CAD build for the part. Positions are in the model's coordinates, mm. Face numbers are marked on the shaded views. A direction names the side the tool comes from. Round coordinates to 2 decimals unless told otherwise and drop trailing zeros. Loops run counter-clockwise (first coordinate to the right, second up) from the corner with the lowest first, then second, coordinate; pieces in that order, holes last.
Autodesk Inventor part; units mm, degrees
ref_plane "Start plane" through (0, 0, 15.875) normal (0, 0, 1) x (1, 0, 0)
ref_plane "End plane" through (0, 0, 98.425) normal (0, 0, 1) x (1, 0, 0)
ref_plane "Work Plane4" through (-9.525, 101.6003, 15.875) normal (0, 0, -1) x (-1, 0, 0)
ref_plane "Start plane" through (0, 0, 15.875) normal (0, 0, 1) x (1, 0, 0)
ref_plane "End plane" through (0, 0, 98.425) normal (0, 0, 1) x (1, 0, 0)
sketch "Sketch" plane through (0, 0, 0) normal (0, 0, 1) x (1, 0, 0)
  line L0 (-15.875, -9.525) -> (-15.875, 9.525)
  line L1 (-9.525, 15.875) -> (9.525, 15.875)
  line L2 (15.875, 9.525) -> (15.875, -9.525)
  line L3 (9.525, -15.875) -> (-9.525, -15.875)
  arc A0 (-15.875, -9.525) -> (-9.525, -15.875) centre (-9.525, -9.525) ccw
  arc A1 (-9.525, 15.875) -> (-15.875, 9.525) centre (-9.525, 9.525) ccw
  arc A2 (15.875, 9.525) -> (9.525, 15.875) centre (9.525, 9.525) ccw
  arc A3 (9.525, -15.875) -> (15.875, -9.525) centre (9.525, -9.525) ccw
  arc A4 (-9.525, 12.7) -> (-12.7, 9.525) centre (-9.525, 9.525) ccw
  line L4 (-9.525, 12.7) -> (9.525, 12.7)
  arc A5 (12.7, 9.525) -> (9.525, 12.7) centre (9.525, 9.525) ccw
  line L5 (12.7, 9.525) -> (12.7, -9.525)
  arc A6 (9.525, -12.7) -> (12.7, -9.525) centre (9.525, -9.525) ccw
  line L6 (9.525, -12.7) -> (-9.525, -12.7)
  arc A7 (-12.7, -9.525) -> (-9.525, -12.7) centre (-9.525, -9.525) ccw
  line L7 (-12.7, -9.525) -> (-12.7, 9.525)
  line L8 (0, 24.0662) -> (0, -24.0662) construction
  line L9 (-24.0662, 0) -> (24.0662, 0) construction
  dimension "d10" = 31.75
  dimension "d11" = 31.75
  dimension "d12" = 3.175
  dimension "d15" = 15.875
  dimension "d16" = 15.875
  dimension "d17" = 6.35
extrude "Body" add sketch "Sketch" along normal up to surface (82.55 mm away) from surface at 15.875
sketch "Sketch3" plane through (0, 0, 0) normal (0, 0, 1) x (1, 0, 0)
  line L0 (0, 0) -> (10, 0)
ref_plane "Work Plane3" through (0, 0, 0) normal (0, -1, 0) x (1, 0, 0)
sketch "Sketch4" plane through (0, 0, 0) normal (0, -1, 0) x (1, 0, 0)
  line L0 (-2, 15.875) -> (12, 15.875)
  line L1 (-2, 98.425) -> (12, 98.425)
  dimension "d19" = 82.55
ref_plane "Work Plane4" through (-9.525, 101.6003, 15.875) normal (0, 0, -1) x (-1, 0, 0)
split "Split1" plane through (-9.525, 101.6003, 15.875) removes the side toward (0, 0, -1)
ref_plane "Work Plane5" through (9.525, 101.6003, 98.425) normal (0, 0, 1) x (1, 0, 0)
split "Split2" plane through (9.525, 101.6003, 98.425) removes the side toward (0, 0, 1)
equation "\"d10\" = G_H"
equation "\"d11\" = G_W"
equation "\"d12\" = G_T"
equation "\"d15\" = 0.5 * d10"
equation "\"d16\" = 0.5 * d11"
equation "\"d17\" = G_IR"
equation "\"d3\" = G_L"
equation "\"G_W\" = 31.75"
equation "\"G_H\" = 31.75"
equation "\"G_T\" = 3.175"
equation "\"G_IR\" = 6.35"
equation "\"G_L\" = d19"
equation "\"G_OFFSET_START\" = -15.875"
equation "\"G_OFFSET_END\" = -15.875"
equation "\"d13\" = -G_OFFSET_START"
equation "\"d14\" = G_OFFSET_END + B_L"
equation "\"B_L\" = 114.3"
properties part number "AISC HSS - 1-1/4x1-1/4x1/8 - 3.25" material "Steel, Mild"
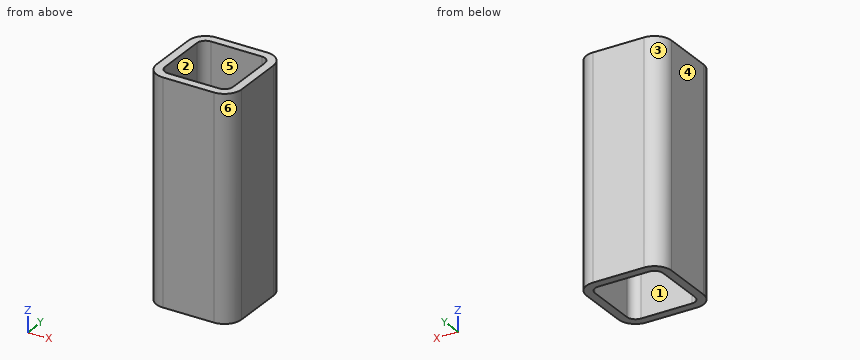
Item 1: Mould opens along Y. For the marked faces 1, 2, 3 and 4 say: released by +Y, released by -Y, zero draft, split by the parting line, or undercut.
Verdict:
face 1: undercut
face 2: undercut
face 3: released by +Y
face 4: zero draft
Item 2: Flat gauge pins, fed straight in: P1, Ø2, axis at x = -12, z = 60, coming from the -Y side; P2, Ø3, axis at y = -12, z = 63, coming from the +X side; P3, Ø4, axis at y = 12, z = 83, coming from the -X side; P4, Ø3, axis at x = 8, y = -10.5, coming from the +Z side. Where does each tip first touch, or does it go through?
Verdict:
P1: stops at y = -15.7
P2: stops at x = 15.8
P3: stops at x = -15.86
P4: passes through
Item 3: Cut at B-B (x = -11.5). List the corners of the cut face in (y, z) (3 decimals).
Verdict:
outline: (-15.56, 15.875) - (-12.011, 15.875) - (-12.011, 98.425) - (-15.56, 98.425) - close; (12.011, 15.875) - (15.56, 15.875) - (15.56, 98.425) - (12.011, 98.425) - close
Item 4: 3-axis set-ups, long thin cutter, end or side, ignore diameter. For the marked faces 5 and 6: which of +Z, -Z, +X, -X, +Y, -Y reach the whole face in a straight line?
Verdict:
face 5: +Z, -Z
face 6: +Z, -Z, +X, -Y
Item 5: Cut at C-C (z = 60). List the corners of the cut face in (x, y) (3 decimals), plus the area to 3 significant figures.
Verdict:
outline: (-15.875, -9.525) arc R6.35 ccw to (-9.525, -15.875) - (9.525, -15.875) arc R6.35 ccw to (15.875, -9.525) - (15.875, 9.525) arc R6.35 ccw to (9.525, 15.875) - (-9.525, 15.875) arc R6.35 ccw to (-15.875, 9.525) - close; hole (-12.7, -9.525) arc R3.175 ccw to (-9.525, -12.7) - (9.525, -12.7) arc R3.175 ccw to (12.7, -9.525) - (12.7, 9.525) arc R3.175 ccw to (9.525, 12.7) - (-9.525, 12.7) arc R3.175 ccw to (-12.7, 9.525) - close
area: 337 mm2
Item 6: Cut at A-A (y = 3). List the corners of the cut face in (x, z) (3 decimals).
Verdict:
outline: (-15.875, 15.875) - (-12.7, 15.875) - (-12.7, 98.425) - (-15.875, 98.425) - close; (12.7, 15.875) - (15.875, 15.875) - (15.875, 98.425) - (12.7, 98.425) - close
Item 7: Wall check: L1, parallel to Y at x = -1.5, z = 47 (3 decimals); L2, parallel to Y at x = -11, z = 52. Give the ranges that are in metal, low to high.
Verdict:
L1: y = -15.875 to -12.7, 12.7 to 15.875
L2: y = -15.7 to -12.34, 12.34 to 15.7
